from build123d import *

# Parameters (mm, degrees)
F0_R          = 0.4
F1_DEPTH      = 1.5
F2_DEPTH      = 0.75
F2_DEPTH_BACK = 2.25


# Not quite as in the source:
# - a feature names something its author has since deleted; it is built from what else it names


with BuildPart() as f1:
    # F0 (on Front) → F1 (new body)
    with BuildSketch(Plane.XZ):
        with BuildLine():
            ThreePointArc((-2.2, -2.24940907), (-1.2, -1.24940907), (-2.2, -0.24940907))
            Line((-2.2, -0.24940907), (-4, -0.24940907))
            ThreePointArc((-4, -0.24940907), (-4.8198039027, -1.24940907), (-4, -2.24940907))
            Line((-4, -2.24940907), (-2.2, -2.24940907))
        make_face()
        with BuildLine():
            Line((0, -0.24940907), (-1, -0.24940907))
            Line((-1, -0.24940907), (-2.2, -0.24940907))
            ThreePointArc((-2.2, -0.24940907), (-1.2, -1.24940907), (-2.2, -2.24940907))
            Line((-2.2, -2.24940907), (-1, -2.24940907))
            Line((-1, -2.24940907), (0, -2.24940907))
            ThreePointArc((0, -2.24940907), (1, -1.24940907), (0, -0.24940907))
        make_face()
        with Locations((0, -1.24940907)):
            Circle(F0_R, mode=Mode.SUBTRACT)
        with BuildLine():
            ThreePointArc((-4, -2.24940907), (-4.8198039027, -1.24940907), (-4, -0.24940907))
            Line((-4, -0.24940907), (-6, -0.24940907))
            ThreePointArc((-6, -0.24940907), (-7, -1.24940907), (-6, -2.24940907))
            Line((-6, -2.24940907), (-4, -2.24940907))
        make_face()
        with Locations((-6, -1.24940907)):
            Circle(F0_R, mode=Mode.SUBTRACT)
    extrude(amount=F1_DEPTH)

    # F0 (on Front) → F2 (join, two sides)
    with BuildSketch(Plane.XZ) as f2_sk:
        with BuildLine():
            ThreePointArc((-2.2, -2.24940907), (-1.2, -1.24940907), (-2.2, -0.24940907))
            Line((-2.2, -0.24940907), (-4, -0.24940907))
            ThreePointArc((-4, -0.24940907), (-4.8198039027, -1.24940907), (-4, -2.24940907))
            Line((-4, -2.24940907), (-2.2, -2.24940907))
        make_face()
    extrude(amount=-F2_DEPTH)
    extrude(f2_sk.sketch, amount=F2_DEPTH_BACK)


solid = f1.part
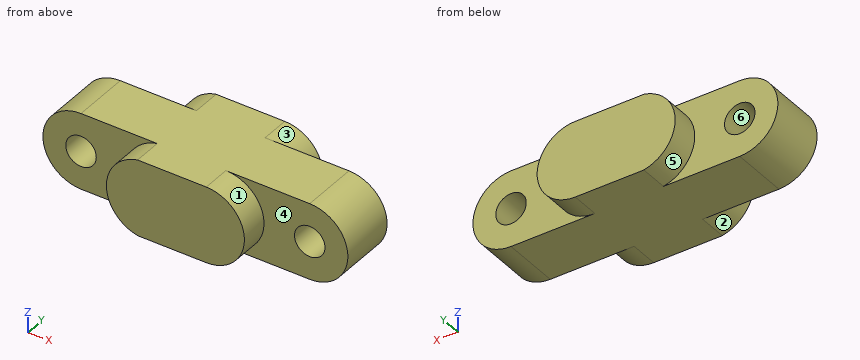
Can you work these out from the model? Positions are in its coordinate system, mm. Face numbers are marked on the shaded views. A direction names the side the tool comes from. Round coordinates to 2 decimals unless told otherwise and drop trailing zeros. Loops run counter-clockwise (first coordinate to the right, second up) from the corner with the lowest first, then second, coordinate; pieces in that order, holes last. Notation, with made-up numbers: (-35.75, -16.75) - (7.25, -16.75) arc R29 ccw to (7.25, 3.25) - close; hole circle Ø1 at (58.5, 86). An arc over 180 degrees is marked (long way). Write item = value, one per line. Start each with the question number.
(1) If we section it at D-D (x = -1.5): Please give me the cut outline in (y, z).
(2) If we section it at C-C (x = -6.25): Please give me the cut outline in (y, z).
(3) If we section it at A-A (z = -1.1): Please give me the cut outline in (x, y).
(4) For the marked faces 1, 2 and 3, which set-ups out of +Z, -Z, +X, -X, +Y, -Y let a thin tool reach every point of the face, with its end or its side?
(5) For P1, Ø0.6, axis at x = -0.5, z = -1.5, coming from the +Y side; P2, Ø0.6, axis at x = -5.5, z = -1, coming from the -Y side, each with a flat end and sliding along its axis, tell me the tip position at first contact or that it passes through.
(6) If we mould it in two halves opening along X, with no side actions, what happens to the marked faces 4, 5 and 6? For each: released by +X, released by -X, zero draft, split by the parting line, or undercut.
(7) If I drill on probe 1 along Z at (x, y) = (0, -0.35); probe 2 along Y at (x, z) = (0.5, -1.7); probe 3 along X at (y, z) = (0.6, -1.25), over which ranges is the centre line in solid material (lowest first)? Write a range as [from, to].
(8) If we section it at B-B (y = -0.75): Please give me the cut outline in (x, z).
Ans:
q1.outline = (-2.25, -1.96) - (-1.5, -1.96) - (-1.5, -2.25) - (0, -2.25) - (0, -1.96) - (0.75, -1.96) - (0.75, -0.54) - (0, -0.54) - (0, -0.25) - (-1.5, -0.25) - (-1.5, -0.54) - (-2.25, -0.54) - close
q2.outline = (-1.5, -2.22) - (0, -2.22) - (0, -1.56) - (-1.5, -1.56) - close; (-1.5, -0.94) - (0, -0.94) - (0, -0.28) - (-1.5, -0.28) - close
q3.outline = (-6.99, -1.5) - (-6.37, -1.5) - (-6.37, 0) - (-6.99, 0) - close; (-5.63, -1.5) - (-4.81, -1.5) - (-4.81, -2.25) - (-1.21, -2.25) - (-1.21, -1.5) - (-0.37, -1.5) - (-0.37, 0) - (-1.21, 0) - (-1.21, 0.75) - (-4.81, 0.75) - (-4.81, 0) - (-5.63, 0) - close; (0.37, -1.5) - (0.99, -1.5) - (0.99, 0) - (0.37, 0) - close
q4.face_1 = +X, -Y
q4.face_2 = -X, -Y
q4.face_3 = +X, +Y
q5.P1 = 0
q5.P2 = -1.5
q6.face_4 = zero draft
q6.face_5 = released by -X
q6.face_6 = undercut
q7.probe_1 = [-2.25, -1.65], [-0.85, -0.25]
q7.probe_2 = [-1.5, 0]
q7.probe_3 = [-4.82, -1.2]
q8.outline = (-6, -2.25) - (0, -2.25) arc R1 ccw to (0, -0.25) - (-6, -0.25) arc R1 ccw to start; hole circle Ø0.8 at (-6, -1.25); hole circle Ø0.8 at (0, -1.25)
